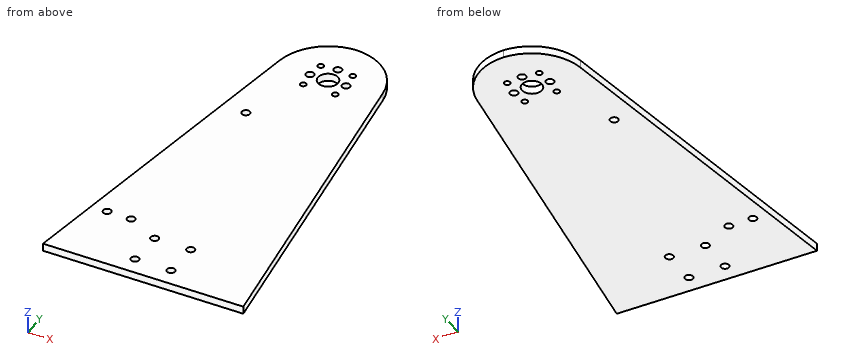
Autodesk Inventor part; units mm, degrees
ref_plane "YZ Plane" through (0, 0, 0) normal (1, 0, 0) x (0, 1, 0)
ref_plane "XZ Plane" through (0, 0, 0) normal (0, 1, 0) x (-1, 0, 0)
ref_plane "XY Plane" through (0, 0, 0) normal (0, 0, 1) x (1, 0, 0)
sketch "Sketch3" plane through (0, 0, 0) normal (0, 0, 1) x (1, 0, 0)
  line L0 (0, 0) -> (100, 0)
  line L1 (100, 0) -> (100, 195) construction
  line L2 (100, 195) -> (0, 195) construction
  line L3 (0, 195) -> (0, 0) construction
  line L4 (50, 0) -> (50, 169) construction
  circle A0 centre (50, 169) radius 4.95
  line L5 (42, 161) -> (58, 161) construction
  line L6 (58, 161) -> (58, 177) construction
  line L7 (58, 177) -> (42, 177) construction
  line L8 (42, 177) -> (42, 161) construction
  line L9 (42, 161) -> (58, 177) construction
  line L10 (58, 161) -> (42, 177) construction
  circle A1 centre (42, 177) radius 1.5
  circle A2 centre (58, 177) radius 1.5
  circle A3 centre (42, 161) radius 1.5
  circle A4 centre (58, 161) radius 1.5
  line L11 (0, 0) -> (24.1871, 172.1)
  line L12 (0, 0) -> (268.3215, 0) construction
  line L13 (100, 0) -> (75.8129, 172.1)
  line L14 (0, 172.1) -> (100, 172.1) construction
  arc A5 (50, 195) -> (24.1871, 172.1) centre (50.5367, 168.3968) ccw
  arc A6 (75.8129, 172.1) -> (50, 195) centre (49.4633, 168.3968) ccw
  line L15 (50, 169) -> (59, 169) construction
  line L16 (50, 169) -> (41, 169) construction
  circle A7 centre (59, 169) radius 2
  circle A8 centre (41, 169) radius 2
  line L17 (41, 9) -> (59, 9) construction
  line L18 (59, 9) -> (59, 27) construction
  line L19 (59, 27) -> (41, 27) construction
  line L20 (41, 27) -> (41, 9) construction
  line L21 (41, 9) -> (59, 27) construction
  line L22 (59, 9) -> (41, 27) construction
  circle A9 centre (41, 27) radius 2
  circle A10 centre (41, 9) radius 2
  circle A11 centre (59, 27) radius 2
  circle A12 centre (59, 9) radius 2
  line L23 (50, 169) -> (50, 178) construction
  circle A13 centre (50, 178) radius 2
  point P0 (37.3431, 265.7102)
  point P1 (62.6569, 265.7102)
  point P2 (50, 18)
  dimension "d3" = 100
  dimension "d4" = 195
  dimension "d5" = 169
  dimension "d6" = 9.9
  dimension "d7" = 16
  dimension "d8" = 16
  dimension "d9" = 3
  dimension "d10" = 3
  dimension "d11" = 3
  dimension "d12" = 3
  dimension "d13" = 82
  dimension "d14" = 22.9
  dimension "d15" = 9
  dimension "d16" = 4
  dimension "d17" = 18
  dimension "d18" = 18
  dimension "d19" = 9
  dimension "d20" = 4
  dimension "d21" = 4
  dimension "d24" = 9
  dimension "d25" = 4
extrude "Extrusion2" add sketch "Sketch3" along normal blind 3.8
sketch "Sketch5" plane through (0, 0, 3.8) normal (0, 0, 1) x (1, 0, 0)
  circle A0 centre (-58.4959, 27.4361) radius 16.3248
  point P0 (0, 0)
sketch "Sketch6" plane through (0, 0, 3.8) normal (0, 0, 1) x (1, 0, 0)
  line L0 (177.5374, 0) -> (-44.6048, 0) construction
  line L1 (173.8282, 35) -> (-48.3141, 35) construction
  circle A0 centre (12.9189, 35) radius 2
  circle A1 centre (24.9189, 35) radius 2
  line L2 (24.1871, 172.1) -> (0, 0)
  point P0 (4.9189, 35)
  dimension "d33" = 35
  dimension "d34" = 4
  dimension "d35" = 4
  dimension "d36" = 12
  dimension "d37" = 8
extrude "Extrusion3" cut sketch "Sketch6" against normal blind 10
sketch "Sketch7" plane through (0, 0, 3.8) normal (0, 0, 1) x (1, 0, 0)
  line L0 (0, 0) -> (115.508, 0) construction
  line L1 (0, 130) -> (115.508, 130)
  line L2 (24.1871, 172.1) -> (0, 0)
  circle A0 centre (30.2703, 130) radius 2
  point P0 (18.2703, 130)
  dimension "d40" = 130
  dimension "d41" = 4
  dimension "d42" = 12
extrude "Extrusion4" cut sketch "Sketch7" against normal blind 10
equation "\"d25\" = d16"
properties part number "Columna" material "PMMA Plastic"
Verification items for the finished model (mm, model axes). Coordinates: 2 decimals unless noted, no trailing zeros. Order: outer loops, then holes, each group sorted by start corner. A loop starts at its lowest first (then second) coordinate and runs counter-clockwise, first axis right, second up. Notation, with made-up numbers: M 64.25,88.5 L 107.25,88.5 A36 ccw 107.25,123.5 Z; hole C 31,75.5 d1. An arc over 180 degrees is marked long. Return JSON: item names as keys, results as strings.
1) Gauge pin test, flat ends, axial feed: pin 1 (2.5 mm diameter, centred on x = 42, y = 177, fed in from +Z); pin 2 (2 mm diameter, centred on y = 121, z = 1, fed in from -X); pin 3 (2 mm diameter, centred on y = 25, z = 1, fed in from +X). Record the tip position at first contact, or that the pin passes through.
Answer list:
{"pin 1": "through", "pin 2": "x = 16.86", "pin 3": "x = 96.63"}
2) Thickness scan on L1, parallel to Y at x = 50, z = 1.25; L2, parallel to X at y = 26.5, z = 2.85; L3, parallel to Y at x = 59, z = 1.9. Record the ranges inside material, lowest first. Write a range as [from, to].
Answer list:
{"L1": "[0, 164.05], [173.95, 176], [180, 195]", "L2": "[3.72, 39.06], [42.94, 57.06], [60.94, 96.28]", "L3": "[0, 7], [11, 25], [29, 159.88], [162.12, 167], [171, 175.88], [178.12, 193.24]"}
3) Cross-section at B-B, the plane y = 9. Record the boundary of the cut face in (x, z), and give its area (3 significant figures).
Answer list:
{"outline": "M 1.26,0 L 39,0 L 39,3.8 L 1.26,3.8 Z; M 43,0 L 57,0 L 57,3.8 L 43,3.8 Z; M 61,0 L 98.74,0 L 98.74,3.8 L 61,3.8 Z", "area": "340 mm2"}
4) Cross-section at C-C, the plane y = 169. Record the boundary of the cut face in (x, z), and give its area (3 significant figures).
Answer list:
{"outline": "M 23.75,0 L 39,0 L 39,3.8 L 23.75,3.8 Z; M 43,0 L 45.05,0 L 45.05,3.8 L 43,3.8 Z; M 54.95,0 L 57,0 L 57,3.8 L 54.95,3.8 Z; M 61,0 L 76.25,0 L 76.25,3.8 L 61,3.8 Z", "area": "131 mm2"}
5) Cross-section at A-A, the plane z = 0.7. Count the separate pieces of the cut face and the enclosed holes in it, and give its area (3 significant figures).
Answer list:
{"separate pieces": "1", "enclosed holes": "15", "area": "13,700 mm2"}
6) Cross-section at D-D, the plane y = 35. Record the boundary of the cut face in (x, z), and give its area (3 significant figures).
Answer list:
{"outline": "M 4.92,0 L 10.92,0 L 10.92,3.8 L 4.92,3.8 Z; M 14.92,0 L 22.92,0 L 22.92,3.8 L 14.92,3.8 Z; M 26.92,0 L 95.08,0 L 95.08,3.8 L 26.92,3.8 Z", "area": "312 mm2"}
